Design review of the part built by this model. Coordinates are the model's own, in mm. Face numbers are marked on the shaded views. A direction names the side the tool comes from. Round coordinates to 2 decimals unless told otherwise and drop trailing zeros. Order: outer loops, then holes, each group sorted by start corner. A loop starts at its lowest first (then second) coordinate and runs counter-clockwise, first axis right, second up. Notation, with made-up numbers: (-33.75, 29) - (11.25, 29) arc R27 ccw to (11.25, 57) - close; hole circle Ø4 at (-34, -2.75). An arc over 180 degrees is marked (long way). Use CSV: the item, a comma, the result in double quotes.
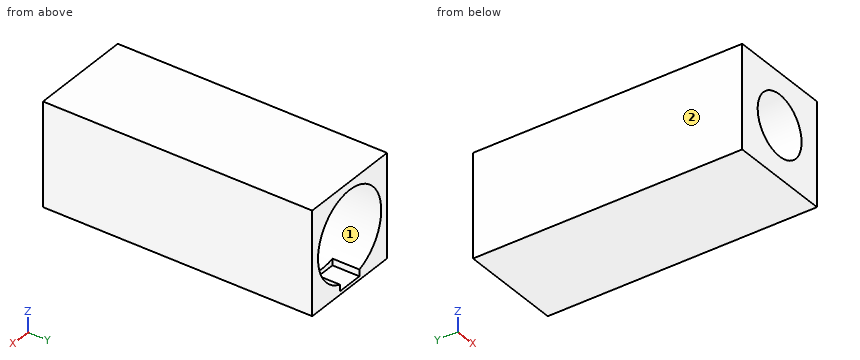
from build123d import *

# Parameters (mm, degrees)
SKETCH1_W           = 23
SKETCH1_H           = 23
BOSS_EXTRUDE1_DEPTH = 60
SKETCH2_R           = 9.725
CUT_EXTRUDE1_DEPTH  = 39
SKETCH3_R           = 6.75
CUT_EXTRUDE2_DEPTH  = 51.783855702
SKETCH5_W           = 6
SKETCH5_H           = 2.398717271
CUT_EXTRUDE3_DEPTH  = 6


with BuildPart() as part:
    # Sketch1 → Boss-Extrude1 (new body)
    with BuildSketch(Plane(origin=(0, 0, 0), x_dir=(-1, 0, 0), z_dir=(0, 1, 0))):
        with Locations((11.5, 11.5)):
            Rectangle(SKETCH1_W, SKETCH1_H)
    extrude(amount=BOSS_EXTRUDE1_DEPTH)

    # Sketch2 → Cut-Extrude1 (cut)
    with BuildSketch(Plane(origin=(0, 60, 0), x_dir=(-1, 0, 0), z_dir=(0, 1, 0))):
        with Locations(Location((11.5, 11.5, 0), (0, 0, 90))):
            Circle(SKETCH2_R)
    extrude(amount=-CUT_EXTRUDE1_DEPTH, mode=Mode.SUBTRACT)

    # Sketch3 → Cut-Extrude2 (cut, through all)
    with BuildSketch(Plane(origin=(0, 21, 0), x_dir=(-1, 0, 0), z_dir=(0, 1, 0))):
        with Locations(Location((11.5, 11.5, 0), (0, 0, 90))):
            Circle(SKETCH3_R)
    extrude(amount=-CUT_EXTRUDE2_DEPTH, mode=Mode.SUBTRACT)

    # Sketch5 → Cut-Extrude3 (cut)
    with BuildSketch(Plane(origin=(0, 60, 0), x_dir=(-1, 0, 0), z_dir=(0, 1, 0))):
        with Locations((11.5, 1.974358636)):
            Rectangle(SKETCH5_W, SKETCH5_H)
    extrude(amount=-CUT_EXTRUDE3_DEPTH, mode=Mode.SUBTRACT)


solid = part.part
1) To check wall thickness, follow L1, parallel to X at y = 31.5, z = 11.5 (3 decimals); L2, parallel to Z at x = -11.5, y = 38 (3 decimals); L3, parallel to Z at x = -6.5, y = 20. State the ranges of each line that lie inside material, in increasing order. Write a range as from..to.
Data:
L1,"x = -23..-21.225, -1.775..0"
L2,"z = 0..1.775, 21.225..23"
L3,"z = 0..6.97, 16.03..23"
2) We need section C-C (z = 11.5). Give the boundary of the cut face in (x, y) (3 decimals), then the cut area to 3 significant figures.
Data:
outline,"(-23, 0) - (-18.25, 0) - (-18.25, 21) - (-21.225, 21) - (-21.225, 60) - (-23, 60) - close; (-4.75, 0) - (0, 0) - (0, 60) - (-1.775, 60) - (-1.775, 21) - (-4.75, 21) - close"
area,"338 mm2"
3) For the marked faces 1 and 2, list the 3-axis set-ups (+Z, -Z, +X, -X, +Y, -Y) from which the entire face can be reached by the end or side of a thin tool; tool diameter is ignored.
Data:
face 1,"+Y"
face 2,"+Z, -Z, -X, +Y, -Y"
4) We need section D-D (x = -3.75). Give the boundary of the cut face in (y, z), then the cut area to 3 significant figures.
Data:
outline,"(0, 0) - (60, 0) - (60, 5.63) - (21, 5.63) - (21, 17.37) - (60, 17.37) - (60, 23) - (0, 23) - close"
area,"922 mm2"
5) We need section B-B (y = 8.5). Give the boundary of the cut face in (x, z), then the cut area to 3 significant figures.
Data:
outline,"(-23, 0) - (0, 0) - (0, 23) - (-23, 23) - close; hole circle Ø13.5 at (-11.5, 11.5)"
area,"386 mm2"
6) Insertion check: pin 1 Ø9.5 at (x, z) = (-10, 8.5) entering from +Y; pin 2 Ø0.7 at (x, z) = (-13, 1.5) entering from +Y. Each pin has a flat end and moves straight along its axis. Give the tip position at first contact, or say it passes through.
Data:
pin 1,"stops at y = 21"
pin 2,"stops at y = 54"
7) We need section A-A (x = -11.5). Give the boundary of the cut face in (y, z) (3 decimals).
Data:
outline,"(0, 0) - (60, 0) - (60, 0.775) - (54, 0.775) - (54, 1.775) - (21, 1.775) - (21, 4.75) - (0, 4.75) - close; (0, 18.25) - (21, 18.25) - (21, 21.225) - (60, 21.225) - (60, 23) - (0, 23) - close"
